Geometry check sheet. Reference: the model listing, model coordinates, mm. Face numbers are marked on the shaded views. A direction names the side the tool comes from. Coordinates: 2 decimals unless noted, no trailing zeros. Order: outer loops, then holes, each group sorted by start corner. A loop starts at its lowest first (then second) coordinate and runs counter-clockwise, first axis right, second up. Notation, with made-up numbers: (63.25, 32.5) -> (71.25, 32.5) arc R16 ccw to (71.25, 61.5) -> close; hole circle Ø5 at (-3.75, -27). An arc over 180 degrees is marked (long way). Answer in a Markdown table with one row per item. Add a question column.
```python
from build123d import *

# Parameters (mm, degrees)
EXTRUDE_1_DEPTH = 137
EXTRUDE_START   = -14.4
EXTRUDE_2_DEPTH = 10
EXTRUDE_START_2 = -114
EXTRUDE_3_DEPTH = 10


with BuildPart() as part:
    # 스케치1 → 보스-돌출1 (new body)
    with BuildSketch(Plane.YZ):
        with BuildLine():
            Line((-16, 19), (16, 19))
            ThreePointArc((16, 19), (18.121320344, 18.121320344), (19, 16))
            Line((19, 16), (19, -16))
            ThreePointArc((19, -16), (18.121320344, -18.121320344), (16, -19))
            Line((16, -19), (-16, -19))
            ThreePointArc((-16, -19), (-18.121320344, -18.121320344), (-19, -16))
            Line((-19, -16), (-19, 16))
            ThreePointArc((-19, 16), (-18.121320344, 18.121320344), (-16, 19))
        make_face()
    extrude(amount=EXTRUDE_1_DEPTH)

    # 스케치2 → 보스-돌출2 (add)
    with BuildSketch(Plane(origin=(0, 0, 0), x_dir=(0, -1, 0), z_dir=(-1, 0, 0)).offset(EXTRUDE_START)):
        with BuildLine():
            Line((-20, 23), (20, 23))
            ThreePointArc((20, 23), (22.121320344, 22.121320344), (23, 20))
            Line((23, 20), (23, -20))
            ThreePointArc((23, -20), (22.121320344, -22.121320344), (20, -23))
            Line((20, -23), (-20, -23))
            ThreePointArc((-20, -23), (-22.121320344, -22.121320344), (-23, -20))
            Line((-23, -20), (-23, 20))
            ThreePointArc((-23, 20), (-22.121320344, 22.121320344), (-20, 23))
        make_face()
    extrude(amount=-EXTRUDE_2_DEPTH)

    # 스케치2<2> → 보스-돌출3 (add)
    with BuildSketch(Plane(origin=(0, 0, 0), x_dir=(0, -1, 0), z_dir=(-1, 0, 0)).offset(EXTRUDE_START_2)):
        with BuildLine():
            Line((-20, 23), (20, 23))
            ThreePointArc((20, 23), (22.121320344, 22.121320344), (23, 20))
            Line((23, 20), (23, -20))
            ThreePointArc((23, -20), (22.121320344, -22.121320344), (20, -23))
            Line((20, -23), (-20, -23))
            ThreePointArc((-20, -23), (-22.121320344, -22.121320344), (-23, -20))
            Line((-23, -20), (-23, 20))
            ThreePointArc((-23, 20), (-22.121320344, 22.121320344), (-20, 23))
        make_face()
    extrude(amount=-EXTRUDE_3_DEPTH)


solid = part.part
```
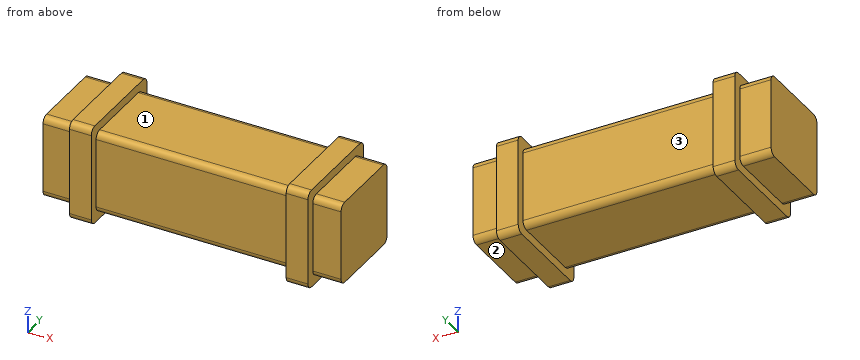
(1) Go/stop test with flat-tipped pins: P1, Ø7, axis at x = 4, z = 5.5, coming from the +Y side; P2, Ø16, axis at x = 5, z = -6, coming from the -Y side; P3, Ø10.5, axis at x = 133, y = -2.5, coming from the -Z side. Record where each tip stops, or that it passes through.
(2) Cross-section at A-A (x = 91). Enter the section's corners in (y, z), plus the area to 3 significant figures.
(3) Cross-section at B-B (z = -4). Enter the section's corners in (x, y), plus the area to 3 significant figures.
(4) Scan lines: line 1 along X through (y, z) = (5.5, 20.5); line 2 along Z through (x, y) = (27.5, 6.5). Record each from-to range of solid material in increasing order.
(5) Access from +Z, -Z, +X, -X, +Y, -Y to the whole of each face (thin tool, end or side, straight path). Record for the marked faces 1, 2 and 3.
Checks:
| question | item | result |
|---|---|---|
| 1 | P1 | y = 19 |
| 1 | P2 | y = -19 |
| 1 | P3 | z = -19 |
| 2 | outline | (-19, -16) arc R3 ccw to (-16, -19) -> (16, -19) arc R3 ccw to (19, -16) -> (19, 16) arc R3 ccw to (16, 19) -> (-16, 19) arc R3 ccw to (-19, 16) -> close |
| 2 | area | 1,440 mm² |
| 3 | outline | (0, -19) -> (14.4, -19) -> (14.4, -23) -> (24.4, -23) -> (24.4, -19) -> (114, -19) -> (114, -23) -> (124, -23) -> (124, -19) -> (137, -19) -> (137, 19) -> (124, 19) -> (124, 23) -> (114, 23) -> (114, 19) -> (24.4, 19) -> (24.4, 23) -> (14.4, 23) -> (14.4, 19) -> (0, 19) -> close |
| 3 | area | 5,370 mm² |
| 4 | line 1 | 14.4 to 24.4, 114 to 124 |
| 4 | line 2 | -19 to 19 |
| 5 | face 1 | +Z, +Y, -Y |
| 5 | face 2 | -Z, +X, +Y, -Y |
| 5 | face 3 | +Z, -Z, +Y |
